The listing builds one solid part. Answer for the finished solid, in the listing's coordinates (mm). A direction names the side the tool comes from. Give positions to 0.01 mm unless a question says otherwise; leave off trailing zeros. Write each loop counter-clockwise with the first axis right and the second up, starting at its lowest first coordinate (ties: lowest second). Pieces come first, ordered by that corner, then holes. Notation, with made-up numbers: M -4.75,-23.75 L 26.25,-23.75 A18 ccw 26.25,-7.75 Z; hole C 31.5,37 d1. An arc over 180 degrees is marked long. Return JSON: item names as keys, results as strings.
from build123d import *

# Parameters (mm, degrees)
ESBO_O1_W                = 97
ESBO_O1_H                = 50
RESSALTO_EXTRUS_O1_DEPTH = 3
CORTE_EXTRUS_O1_REACH    = 56.647
ESBO_O2_W                = 10.782222222
ESBO_O2_H                = 3
CORTE_EXTRUS_O2_REACH    = 56.647
ESBO_O4_W                = 3
ESBO_O4_H                = 10


with BuildPart() as part:
    # Esboço1 → Ressalto-extrusão1 (new body)
    with BuildSketch(Plane(origin=(0, 0, 0), x_dir=(0, 0, -1), z_dir=(1, 0, 0))):
        Rectangle(ESBO_O1_W, ESBO_O1_H)
    extrude(amount=RESSALTO_EXTRUS_O1_DEPTH)

    # Esboço2 → Corte-extrusão1 (cut, up to next)
    with BuildSketch(Plane.ZY, mode=Mode.PRIVATE) as corte_extrus_o1_sk1:
        with Locations((-10.771111111, 23.5)):
            Rectangle(ESBO_O2_W, ESBO_O2_H)
    corte_extrus_o1_tool1 = extrude(corte_extrus_o1_sk1.sketch, amount=-CORTE_EXTRUS_O1_REACH, mode=Mode.PRIVATE) & part.part
    # Esboço2 → Corte-extrusão1 (cut, up to next)
    with BuildSketch(Plane.ZY, mode=Mode.PRIVATE) as corte_extrus_o1_sk2:
        with Locations((-32.331111111, 23.5)):
            Rectangle(ESBO_O2_W, ESBO_O2_H)
    corte_extrus_o1_tool2 = extrude(corte_extrus_o1_sk2.sketch, amount=-CORTE_EXTRUS_O1_REACH, mode=Mode.PRIVATE) & part.part
    # Esboço2 → Corte-extrusão1 (cut, up to next)
    with BuildSketch(Plane.ZY, mode=Mode.PRIVATE) as corte_extrus_o1_sk3:
        with Locations((10.788888889, 23.5)):
            Rectangle(ESBO_O2_W, ESBO_O2_H)
    corte_extrus_o1_tool3 = extrude(corte_extrus_o1_sk3.sketch, amount=-CORTE_EXTRUS_O1_REACH, mode=Mode.PRIVATE) & part.part
    # Esboço2 → Corte-extrusão1 (cut, up to next)
    with BuildSketch(Plane.ZY, mode=Mode.PRIVATE) as corte_extrus_o1_sk4:
        with Locations((32.348888889, 23.5)):
            Rectangle(ESBO_O2_W, ESBO_O2_H)
    corte_extrus_o1_tool4 = extrude(corte_extrus_o1_sk4.sketch, amount=-CORTE_EXTRUS_O1_REACH, mode=Mode.PRIVATE) & part.part
    # Esboço2 → Corte-extrusão1 (cut, up to next)
    with BuildSketch(Plane.ZY, mode=Mode.PRIVATE) as corte_extrus_o1_sk5:
        with Locations((-32.331111111, -23.5)):
            Rectangle(ESBO_O2_W, ESBO_O2_H)
    corte_extrus_o1_tool5 = extrude(corte_extrus_o1_sk5.sketch, amount=-CORTE_EXTRUS_O1_REACH, mode=Mode.PRIVATE) & part.part
    # Esboço2 → Corte-extrusão1 (cut, up to next)
    with BuildSketch(Plane.ZY, mode=Mode.PRIVATE) as corte_extrus_o1_sk6:
        with Locations((32.348888889, -23.5)):
            Rectangle(ESBO_O2_W, ESBO_O2_H)
    corte_extrus_o1_tool6 = extrude(corte_extrus_o1_sk6.sketch, amount=-CORTE_EXTRUS_O1_REACH, mode=Mode.PRIVATE) & part.part
    # Esboço2 → Corte-extrusão1 (cut, up to next)
    with BuildSketch(Plane.ZY, mode=Mode.PRIVATE) as corte_extrus_o1_sk7:
        with Locations((-10.771111111, -23.5)):
            Rectangle(ESBO_O2_W, ESBO_O2_H)
    corte_extrus_o1_tool7 = extrude(corte_extrus_o1_sk7.sketch, amount=-CORTE_EXTRUS_O1_REACH, mode=Mode.PRIVATE) & part.part
    # Esboço2 → Corte-extrusão1 (cut, up to next)
    with BuildSketch(Plane.ZY, mode=Mode.PRIVATE) as corte_extrus_o1_sk8:
        with Locations((10.788888889, -23.5)):
            Rectangle(ESBO_O2_W, ESBO_O2_H)
    corte_extrus_o1_tool8 = extrude(corte_extrus_o1_sk8.sketch, amount=-CORTE_EXTRUS_O1_REACH, mode=Mode.PRIVATE) & part.part
    add(corte_extrus_o1_tool1.solids().sort_by_distance((0, 23.5, -10.771111))[0], mode=Mode.SUBTRACT)
    add(corte_extrus_o1_tool2.solids().sort_by_distance((0, 23.5, -32.331111))[0], mode=Mode.SUBTRACT)
    add(corte_extrus_o1_tool3.solids().sort_by_distance((0, 23.5, 10.788889))[0], mode=Mode.SUBTRACT)
    add(corte_extrus_o1_tool4.solids().sort_by_distance((0, 23.5, 32.348889))[0], mode=Mode.SUBTRACT)
    add(corte_extrus_o1_tool5.solids().sort_by_distance((0, -23.5, -32.331111))[0], mode=Mode.SUBTRACT)
    add(corte_extrus_o1_tool6.solids().sort_by_distance((0, -23.5, 32.348889))[0], mode=Mode.SUBTRACT)
    add(corte_extrus_o1_tool7.solids().sort_by_distance((0, -23.5, -10.771111))[0], mode=Mode.SUBTRACT)
    add(corte_extrus_o1_tool8.solids().sort_by_distance((0, -23.5, 10.788889))[0], mode=Mode.SUBTRACT)

    # Esboço4 → Corte-extrusão2 (cut, up to next)
    with BuildSketch(Plane.ZY, mode=Mode.PRIVATE) as corte_extrus_o2_sk1:
        with Locations((47, 20)):
            Rectangle(ESBO_O4_W, ESBO_O4_H)
    corte_extrus_o2_tool1 = extrude(corte_extrus_o2_sk1.sketch, amount=-CORTE_EXTRUS_O2_REACH, mode=Mode.PRIVATE) & part.part
    # Esboço4 → Corte-extrusão2 (cut, up to next)
    with BuildSketch(Plane.ZY, mode=Mode.PRIVATE) as corte_extrus_o2_sk2:
        with Locations((47, -20)):
            Rectangle(ESBO_O4_W, ESBO_O4_H)
    corte_extrus_o2_tool2 = extrude(corte_extrus_o2_sk2.sketch, amount=-CORTE_EXTRUS_O2_REACH, mode=Mode.PRIVATE) & part.part
    # Esboço4 → Corte-extrusão2 (cut, up to next)
    with BuildSketch(Plane.ZY, mode=Mode.PRIVATE) as corte_extrus_o2_sk3:
        with Locations((-47, 0)):
            Rectangle(ESBO_O4_W, ESBO_O4_H)
    corte_extrus_o2_tool3 = extrude(corte_extrus_o2_sk3.sketch, amount=-CORTE_EXTRUS_O2_REACH, mode=Mode.PRIVATE) & part.part
    # Esboço4 → Corte-extrusão2 (cut, up to next)
    with BuildSketch(Plane.ZY, mode=Mode.PRIVATE) as corte_extrus_o2_sk4:
        with Locations((-47, 20)):
            Rectangle(ESBO_O4_W, ESBO_O4_H)
    corte_extrus_o2_tool4 = extrude(corte_extrus_o2_sk4.sketch, amount=-CORTE_EXTRUS_O2_REACH, mode=Mode.PRIVATE) & part.part
    # Esboço4 → Corte-extrusão2 (cut, up to next)
    with BuildSketch(Plane.ZY, mode=Mode.PRIVATE) as corte_extrus_o2_sk5:
        with Locations((47, 0)):
            Rectangle(ESBO_O4_W, ESBO_O4_H)
    corte_extrus_o2_tool5 = extrude(corte_extrus_o2_sk5.sketch, amount=-CORTE_EXTRUS_O2_REACH, mode=Mode.PRIVATE) & part.part
    # Esboço4 → Corte-extrusão2 (cut, up to next)
    with BuildSketch(Plane.ZY, mode=Mode.PRIVATE) as corte_extrus_o2_sk6:
        with Locations((-47, -20)):
            Rectangle(ESBO_O4_W, ESBO_O4_H)
    corte_extrus_o2_tool6 = extrude(corte_extrus_o2_sk6.sketch, amount=-CORTE_EXTRUS_O2_REACH, mode=Mode.PRIVATE) & part.part
    add(corte_extrus_o2_tool1.solids().sort_by_distance((0, 20, 47))[0], mode=Mode.SUBTRACT)
    add(corte_extrus_o2_tool2.solids().sort_by_distance((0, -20, 47))[0], mode=Mode.SUBTRACT)
    add(corte_extrus_o2_tool3.solids().sort_by_distance((0, 0, -47))[0], mode=Mode.SUBTRACT)
    add(corte_extrus_o2_tool4.solids().sort_by_distance((0, 20, -47))[0], mode=Mode.SUBTRACT)
    add(corte_extrus_o2_tool5.solids().sort_by_distance((0, 0, 47))[0], mode=Mode.SUBTRACT)
    add(corte_extrus_o2_tool6.solids().sort_by_distance((0, -20, -47))[0], mode=Mode.SUBTRACT)


solid = part.part
Item 1: A cutting plane is placed at B-B, the plane y = -1.5. Write down the section's boundary in (x, z), plus the area to 3 significant figures.
Geometry results:
{"outline": "M 0,-45.5 L 3,-45.5 L 3,45.5 L 0,45.5 Z", "area": "273 mm2"}
Item 2: Find the intervals of material crossed by line 1 (Z direction, x = 0.9, y = -23); line 2 (Y direction, x = 1.65, z = 6); line 3 (Z direction, x = 0.4, y = 21), in increasing order.
Geometry results:
{"line 1": "z = -45.5 to -37.72, -26.94 to -16.16, -5.38 to 5.4, 16.18 to 26.96, 37.74 to 45.5", "line 2": "y = -22 to 22", "line 3": "z = -45.5 to 45.5"}
Item 3: A cutting plane is placed at A-A, the plane z = 7. Write down the section's boundary in (x, y).
Geometry results:
{"outline": "M 0,-22 L 3,-22 L 3,22 L 0,22 Z"}
Item 4: Which of the six approach directions +Z, -Z, +X, -X, +Y, -Y give full straight-line access (tool end or side, diameter ignored) to faces 1 (the flat face through (1, 20, 45.5)), 2 (the flat face through (1, -24, 37.74)), 3 (the flat face through (1, 23, -37.722))?
Geometry results:
{"face 1": "+Z, +X, -X, +Y", "face 2": "+X, -X, -Y", "face 3": "+X, -X, +Y"}
Item 5: Determine the mould class of faces 4 (the flat face through (1, 22, -11)), 5 (the flat face through (1, -24, -26.94)), 6 (the flat face through (1, 5, -47)) for opening direction Y: +Y half, -Y half, draft (parallel to the pull), parting line (faces both ways), or undercut.
Geometry results:
{"face 4": "+Y half", "face 5": "draft", "face 6": "undercut"}
Item 6: Given pin 1 Ø1.5 at (x, y) = (2, -24) entering from -Z; pin 2 Ø0.9 at (x, z) = (1.5, -9.5) entering from +Y; pin 3 Ø1.5 at (x, y) = (2, 19.5) entering from +Z, each flat-ended and moving along its own axis, determine where each tip first touches the part or whether it passes through.
Geometry results:
{"pin 1": "stops at z = -45.5", "pin 2": "stops at y = 22", "pin 3": "stops at z = 45.5"}
